Drawing for the job (mm, zero at the part's lowest x, y, z). Coordinates: 2 decimals unless noted, no trailing zeros. Loops run counter-clockwise (first coordinate to the right, second up) from the corner with the lowest first, then second, coordinate; pieces in that order, holes last. Notation, with made-up numbers: (19, -23) -> (76, -23) arc R26 ccw to (76, 11) -> close; hole circle Ø2 at (53.25, -4.75). An arc over 180 degrees is marked (long way). Write item = value, one per line. Start each with the question number.
(1) Band-saw the part on D-D (z = 27). Write the cut outline in (x, y).
(2) Drill centre lines: line 1 (Y direction, x = 25.4, z = 144) (3 decimals); line 2 (Y direction, x = 177, z = 199); line 3 (Z direction, x = 368.5, y = 60.5). Where is each one in solid material? Low to high. Write a range as from..to.
(3) Band-saw the part on C-C (x = 132). Write the cut outline in (y, z), and give its area (3 significant figures).
(4) Band-saw the part on B-B (y = 29). Write the cut outline in (x, z).
(5) Band-saw the part on A-A (x = 374.65). Write the cut outline in (y, z) (3 decimals).
(6) Flat gauge pins, fed straight in: P1, Ø15, axis at x = 45.5, y = 39, coming from the +Z side; P2, Ø1.5, axis at x = 89.5, z = 136.5, coming from the +Y side. Where does each tip first touch, or does it go through?
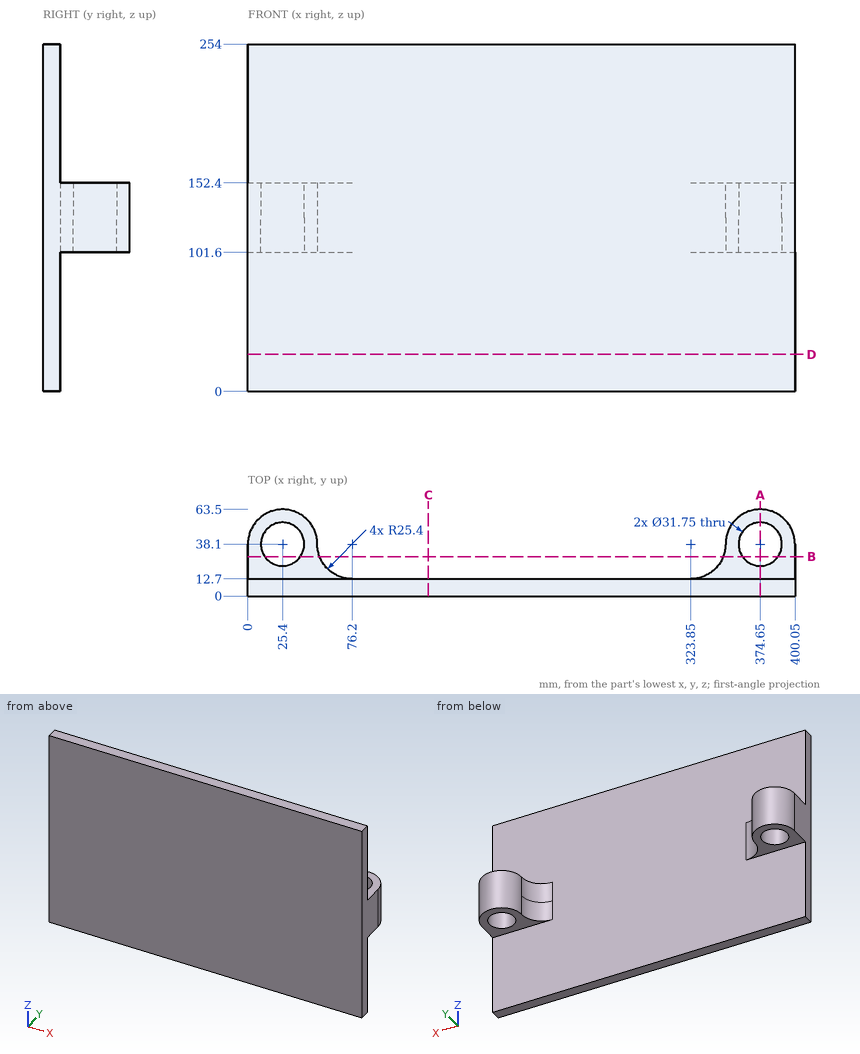
Findings below:
q1.outline = (0, 0) -> (400.05, 0) -> (400.05, 12.7) -> (0, 12.7) -> close
q2.line_1 = 0..22.225, 53.975..63.5
q2.line_2 = 0..12.7
q2.line_3 = 101.6..152.4
q3.outline = (0, 0) -> (12.7, 0) -> (12.7, 254) -> (0, 254) -> close
q3.area = 3,230 mm²
q4.outline = (0, 101.6) -> (12.39, 101.6) -> (12.39, 152.4) -> (0, 152.4) -> close; (38.41, 101.6) -> (52.49, 101.6) -> (52.49, 152.4) -> (38.41, 152.4) -> close; (347.56, 101.6) -> (361.64, 101.6) -> (361.64, 152.4) -> (347.56, 152.4) -> close; (387.66, 101.6) -> (400.05, 101.6) -> (400.05, 152.4) -> (387.66, 152.4) -> close
q5.outline = (0, 0) -> (12.7, 0) -> (12.7, 101.6) -> (22.225, 101.6) -> (22.225, 152.4) -> (12.7, 152.4) -> (12.7, 254) -> (0, 254) -> close; (53.975, 101.6) -> (63.5, 101.6) -> (63.5, 152.4) -> (53.975, 152.4) -> close
q6.P1 = 152.4
q6.P2 = 12.7
